Verification items for the finished model (mm, model axes). A direction names the side the tool comes from. Give positions to 0.01 mm unless a question says otherwise; leave off trailing zeros. Loops run counter-clockwise (first coordinate to the right, second up) from the corner with the lowest first, then second, coordinate; pieces in that order, holes last. Notation, with made-up numbers: M 81,-39.75 L 103,-39.75 A17 ccw 103,-31.75 Z; hole C 23,-39 d11. An arc over 180 degrees is marked long. Use a Markdown table: item, result.
from build123d import *

# Parameters (mm, degrees)
SKETCH_2_W          = 140
SKETCH_2_H          = 140
EXTRUDE_1_DEPTH     = 4
EXTRUDE_1_2_DEPTH   = 100
EXTRUDE_2_DEPTH     = 2
CUT_EXTRUDE_1_DEPTH = 115.5
SKETCH_6_R          = 6.5
CUT_EXTRUDE_2_DEPTH = 5
FILLET_1_R          = 10
CUT_EXTRUDE_3_REACH = 96


with BuildPart() as part:
    # Эскиз2 → Extrude 1 (new body)
    with BuildSketch(Plane(origin=(0, 0, 0), x_dir=(1, 0, 0), z_dir=(0, 1, 0))):
        Rectangle(SKETCH_2_W, SKETCH_2_H)
    extrude(amount=EXTRUDE_1_DEPTH)

    # Эскиз3 → Extrude 1 2 (add)
    with BuildSketch(Plane(origin=(0, 4, 0), x_dir=(1, 0, 0), z_dir=(0, 1, 0))):
        with BuildLine():
            Line((-40.5, -20), (-40.5, 19))
            ThreePointArc((-40.5, 19), (-40.207106781, 19.707106781), (-39.5, 20))
            Line((-39.5, 20), (39.5, 20))
            ThreePointArc((39.5, 20), (40.207106781, 19.707106781), (40.5, 19))
            Line((40.5, 19), (40.5, -20))
            Line((40.5, -20), (44.5, -20))
            Line((44.5, -20), (44.5, 19))
            ThreePointArc((44.5, 19), (43.035533906, 22.535533906), (39.5, 24))
            Line((39.5, 24), (-39.5, 24))
            ThreePointArc((-39.5, 24), (-43.035533906, 22.535533906), (-44.5, 19))
            Line((-44.5, 19), (-44.5, -20))
            Line((-44.5, -20), (-40.5, -20))
        make_face()
    extrude(amount=EXTRUDE_1_2_DEPTH)

    # Эскиз4 → Бобышка-Вытянуть2 (add, symmetric)
    with BuildSketch(Plane(origin=(0, 0, 0), x_dir=(0, 0, -1), z_dir=(1, 0, 0))):
        Polygon((24, 75.01408311), (65, 4), (24, 4), align=None)
    extrude(amount=EXTRUDE_2_DEPTH, both=True)

    # Эскиз5 → Вырез-Вытянуть1 (cut, through all)
    with BuildSketch(Plane(origin=(44.5, 0, 0), x_dir=(0, 0, -1), z_dir=(1, 0, 0))):
        with BuildLine():
            Line((5, 92), (5, 80))
            ThreePointArc((5, 80), (0, 75), (-5, 80))
            Line((-5, 80), (-5, 92))
            ThreePointArc((-5, 92), (0, 97), (5, 92))
        make_face()
        with BuildLine():
            Line((5, 28), (5, 16))
            ThreePointArc((5, 16), (0, 11), (-5, 16))
            Line((-5, 16), (-5, 28))
            ThreePointArc((-5, 28), (0, 33), (5, 28))
        make_face()
    extrude(amount=-CUT_EXTRUDE_1_DEPTH, mode=Mode.SUBTRACT)

    # Эскиз6 → Вырез-Вытянуть2 (cut, through all)
    with BuildSketch(Plane(origin=(0, 4, 0), x_dir=(1, 0, 0), z_dir=(0, 1, 0))):
        with Locations(Location((-55, 55, 0), (0, 0, 270))):  # turned: the seam where the file's is
            Circle(SKETCH_6_R)
        with Locations(Location((-55, -55, 0), (0, 0, 270))):  # turned: the seam where the file's is
            Circle(SKETCH_6_R)
        with Locations(Location((55, 55, 0), (0, 0, 270))):  # turned: the seam where the file's is
            Circle(SKETCH_6_R)
        with Locations(Location((55, -55, 0), (0, 0, 270))):  # turned: the seam where the file's is
            Circle(SKETCH_6_R)
    extrude(amount=-CUT_EXTRUDE_2_DEPTH, mode=Mode.SUBTRACT)

    # Скругление1
    fillet_1_edges = [part.edges().sort_by_distance(p)[0] for p in [
        (70, 2, 70),
        (-70, 2, 70),
        (-70, 2, -70),
        (70, 2, -70),
    ]]
    fillet(fillet_1_edges, radius=FILLET_1_R)

    # Эскиз8 → Вырез-Вытянуть3 (cut, up to next)
    with BuildSketch(Plane(origin=(0, 0, -24), x_dir=(-1, 0, 0), z_dir=(0, 0, -1)), mode=Mode.PRIVATE) as cut_extrude_3_sk1:
        with BuildLine():
            Line((-15, 92), (-15, 80))
            ThreePointArc((-15, 80), (-20, 75), (-25, 80))
            Line((-25, 80), (-25, 92))
            ThreePointArc((-25, 92), (-20, 97), (-15, 92))
        make_face()
    cut_extrude_3_tool1 = extrude(cut_extrude_3_sk1.sketch, amount=-CUT_EXTRUDE_3_REACH, mode=Mode.PRIVATE) & part.part
    add(cut_extrude_3_tool1.solids().sort_by_distance((20, 86, -24))[0], mode=Mode.SUBTRACT)
    # Эскиз8 → Вырез-Вытянуть3 (cut, up to next)
    with BuildSketch(Plane(origin=(0, 0, -24), x_dir=(-1, 0, 0), z_dir=(0, 0, -1)), mode=Mode.PRIVATE) as cut_extrude_3_sk2:
        with BuildLine():
            Line((-15, 28), (-15, 16))
            ThreePointArc((-15, 16), (-20, 11), (-25, 16))
            Line((-25, 16), (-25, 28))
            ThreePointArc((-25, 28), (-20, 33), (-15, 28))
        make_face()
    cut_extrude_3_tool2 = extrude(cut_extrude_3_sk2.sketch, amount=-CUT_EXTRUDE_3_REACH, mode=Mode.PRIVATE) & part.part
    add(cut_extrude_3_tool2.solids().sort_by_distance((20, 22, -24))[0], mode=Mode.SUBTRACT)
    # Эскиз8 → Вырез-Вытянуть3 (cut, up to next)
    with BuildSketch(Plane(origin=(0, 0, -24), x_dir=(-1, 0, 0), z_dir=(0, 0, -1)), mode=Mode.PRIVATE) as cut_extrude_3_sk3:
        with BuildLine():
            Line((15, 92), (15, 80))
            ThreePointArc((15, 80), (20, 75), (25, 80))
            Line((25, 80), (25, 92))
            ThreePointArc((25, 92), (20, 97), (15, 92))
        make_face()
    cut_extrude_3_tool3 = extrude(cut_extrude_3_sk3.sketch, amount=-CUT_EXTRUDE_3_REACH, mode=Mode.PRIVATE) & part.part
    add(cut_extrude_3_tool3.solids().sort_by_distance((-20, 86, -24))[0], mode=Mode.SUBTRACT)
    # Эскиз8 → Вырез-Вытянуть3 (cut, up to next)
    with BuildSketch(Plane(origin=(0, 0, -24), x_dir=(-1, 0, 0), z_dir=(0, 0, -1)), mode=Mode.PRIVATE) as cut_extrude_3_sk4:
        with BuildLine():
            Line((15, 28), (15, 16))
            ThreePointArc((15, 16), (20, 11), (25, 16))
            Line((25, 16), (25, 28))
            ThreePointArc((25, 28), (20, 33), (15, 28))
        make_face()
    cut_extrude_3_tool4 = extrude(cut_extrude_3_sk4.sketch, amount=-CUT_EXTRUDE_3_REACH, mode=Mode.PRIVATE) & part.part
    add(cut_extrude_3_tool4.solids().sort_by_distance((-20, 22, -24))[0], mode=Mode.SUBTRACT)


solid = part.part
(1) Draft check along X on faces 1 (the flat face through (44.5, 53, 1)), 2 (the cylindrical face through (-20, 11, -22)), 3 (the cylindrical face through (-43, 53.3, -22.57)). Enter one of: +X half, -X half, draft (parallel to the pull), parting line (faces both ways), or undercut.
Results below:
| item | result |
|---|---|
| face 1 | +X half |
| face 2 | undercut |
| face 3 | -X half |
(2) Cross-section at C-C on y = 84. Record the cut outline in (x, z), then the cut area to 3 significant figures.
Results below:
| item | result |
|---|---|
| outline | M -44.5,-19 A5 ccw -39.5,-24 L -25,-24 L -25,-20 L -39.5,-20 A1 cw -40.5,-19 L -40.5,-5 L -44.5,-5 Z; M -44.5,5 L -40.5,5 L -40.5,20 L -44.5,20 Z; M -15,-24 L 15,-24 L 15,-20 L -15,-20 Z; M 25,-24 L 39.5,-24 A5 ccw 44.5,-19 L 44.5,-5 L 40.5,-5 L 40.5,-19 A1 cw 39.5,-20 L 25,-20 Z; M 40.5,5 L 44.5,5 L 44.5,20 L 40.5,20 Z |
| area | 506 mm^2 |
(3) Cross-section at D-D on x = -11.5. Record the cut outline in (y, z).
Results below:
| item | result |
|---|---|
| outline | M 0,-70 L 4,-70 L 4,-24 L 104,-24 L 104,-20 L 4,-20 L 4,70 L 0,70 Z |
(4) Set-up check for faces 4 (the cylindrical face through (-67.15, 2.03, 66.99)), 5 (the flat face through (15, 22, -22)), 6 (the flat face through (43, 86, 5)), 7 (the flat face through (-43, 53, 20)), 8 (the flat face through (-40.5, 53, 1)): record each of +Z, -Z, +X, -X, +Y, -Y from which the full face is reachable in a straight line by a thin tool's end or side.
Results below:
| item | result |
|---|---|
| face 4 | +Z, -X, +Y, -Y |
| face 5 | +Z, -Z |
| face 6 | +X, -X |
| face 7 | +Z, +X, -X, +Y |
| face 8 | +Z, +Y |
(5) Cross-section at B-B on x = 20. Record the cut outline in (y, z).
Results below:
| item | result |
|---|---|
| outline | M 0,-70 L 4,-70 L 4,-24 L 11,-24 L 11,-20 L 4,-20 L 4,70 L 0,70 Z; M 33,-24 L 75,-24 L 75,-20 L 33,-20 Z; M 97,-24 L 104,-24 L 104,-20 L 97,-20 Z |
(6) Gauge pin test, flat ends, axial feed: P1, Ø4, axis at x = -28.5, z = 17.5, coming from the +Y side; P2, Ø4.5, axis at y = 24.5, z = -22.5, coming from the +X side; P3, Ø1.2, axis at x = 43, y = 20.5, coming from the +Z side; P4, Ø2, axis at x = 53.5, z = 32.5, coming from the -Y side. Record the tip position at first contact, or that the pin passes through.
Results below:
| item | result |
|---|---|
| P1 | y = 4 |
| P2 | x = 44.34 |
| P3 | z = 20 |
| P4 | y = 0 |
(7) Cross-section at A-A on z = 0. Record the cut outline in (x, y), then the cut area to 3 significant figures.
Results below:
| item | result |
|---|---|
| outline | M -70,0 L 70,0 L 70,4 L 44.5,4 L 44.5,11 L 40.5,11 L 40.5,4 L -40.5,4 L -40.5,11 L -44.5,11 L -44.5,4 L -70,4 Z; M -44.5,33 L -40.5,33 L -40.5,75 L -44.5,75 Z; M -44.5,97 L -40.5,97 L -40.5,104 L -44.5,104 Z; M 40.5,33 L 44.5,33 L 44.5,75 L 40.5,75 Z; M 40.5,97 L 44.5,97 L 44.5,104 L 40.5,104 Z |
| area | 1,010 mm^2 |
(8) Material ranges on line 1 (X direction, y = 2, z = 55); line 2 (Y direction, x = 62, z = -4.5); line 3 (Z direction, x = -39.5, y = 16.5), recorded low to high.
Results below:
| item | result |
|---|---|
| line 1 | -70 to -61.5, -48.5 to 48.5, 61.5 to 70 |
| line 2 | 0 to 4 |
| line 3 | -24 to -20 |
